Source: CAD feature listing. Evaluate the final solid. Frame: model axes, mm. Coordinates: 2 decimals unless noted, no trailing zeros. Loops run counter-clockwise (first coordinate to the right, second up) from the corner with the lowest first, then second, coordinate; pieces in that order, holes last.
Item 1: Line query: probe 1 along Y at (x, z) = (48.5, 1); probe 2 along Y at (x, z) = (-6.5, 2.75); probe 3 along X at (y, z) = (-107, 3). Output: solid intervals per line, ascending.
Item 2: Section query B-B, the plane y = -98.5. Return the cut outline in (x, z).
Item 3: Section query C-C, the plane x = 37. Return the cut outline in (y, z).
Item 4: Section query A-A, the plane z = 4.75. State how many separate pieces and enclosed holes the cut face has, then the cut area to 3 significant figures.
Item 5: Pin query (flat end, axial travel): pin 1 Ø7.5 at (x, y) = (50.3, -108.65) entering from +Z. Return the tip coordinate at first contact, or that it passes through.
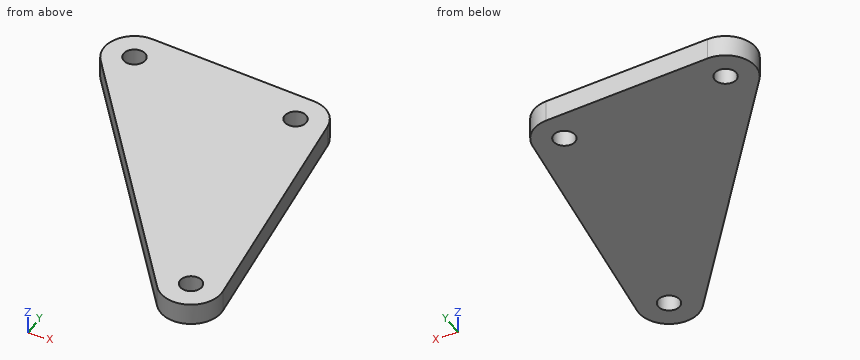
```python
from build123d import *

# Parameters (mm, degrees)
SKETCH1_R           = 3.175
BOSS_EXTRUDE1_DEPTH = 6.35
FILLET1_R           = 8.89


with BuildPart() as part:
    # Sketch1 → Boss-Extrude1 (new body)
    with BuildSketch(Plane.XY):
        Polygon((-26.572670207, -20.693163298), (49.414762795, -26.00204572), (63.045667666, -140.545952681), align=None)
        with Locations((-7.829487562, -30.914331115)):
            Circle(SKETCH1_R, mode=Mode.SUBTRACT)
        with Locations((41.456372883, -34.357700996)):
            Circle(SKETCH1_R, mode=Mode.SUBTRACT)
        with Locations((50.297451581, -108.651499199)):
            Circle(SKETCH1_R, mode=Mode.SUBTRACT)
    extrude(amount=BOSS_EXTRUDE1_DEPTH)

    # Fillet1
    fillet1_edges = [part.edges().sort_by_distance(p)[0] for p in [
        (-26.572670207, -20.693163298, 3.175),
        (49.414762795, -26.00204572, 3.175),
        (63.045667666, -140.545952681, 3.175),
    ]]
    fillet(fillet1_edges, radius=FILLET1_R)


solid = part.part
```
Verdict:
1. probe 1: y = -117.36 to -111.27, -106.03 to -28.93
1. probe 2: y = -47.54 to -33.8, -28.03 to -22.1
1. probe 3: x = 37.96 to 47.59, 53.01 to 59.05
2. outline: (31.61, 0) - (58.04, 0) - (58.04, 6.35) - (31.61, 6.35) - close
3. outline: (-105.71, 0) - (-25.13, 0) - (-25.13, 6.35) - (-105.71, 6.35) - close
4. separate pieces: 1
4. enclosed holes: 3
4. area: 3,940 mm2
5. pin 1: stops at z = 6.35
